Can you work these out from the drawing? Everything is in mm from the part's minimum corner. Round coordinates to 2 decimals unless told otherwise and drop trailing zeros. Order: outer loops, then holes, each group sorted by start corner. A loop starts at its lowest first (then second) coordinate and runs counter-clockwise, first axis right, second up. Notation, with made-up numbers: (74, -21) -> (122, -21) arc R14 cw to (122, 6) -> close; hole circle Ø8 at (12, -1.75). An arc over 180 degrees is marked (long way). One line per item, written item: value.
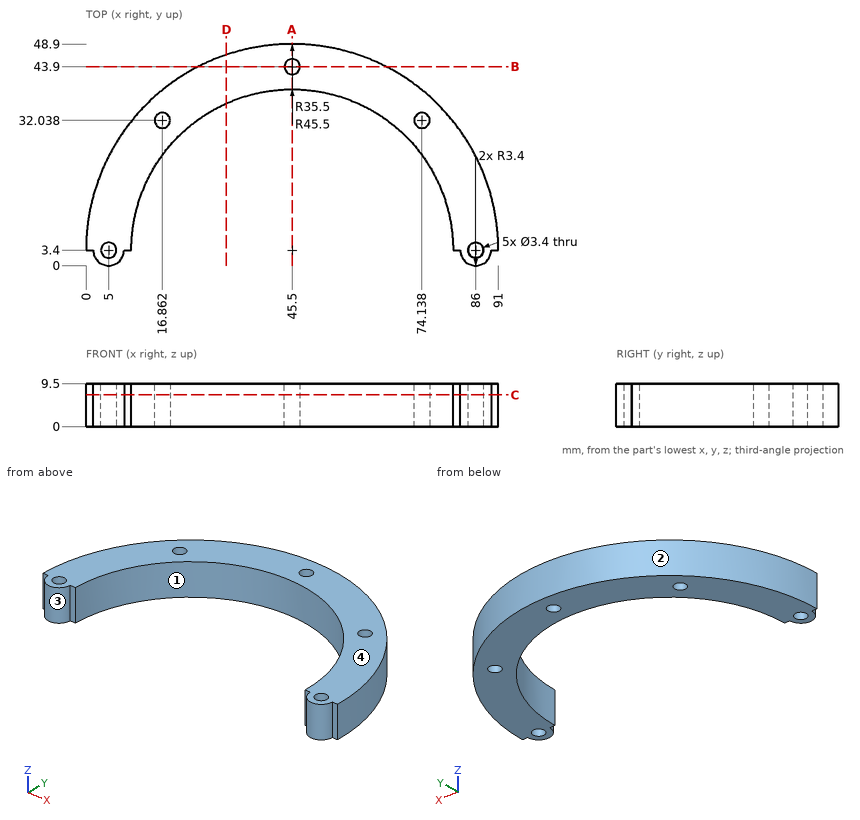
Q1. I want a section at A-A on x = 45.5. List the corners of the cut face in (y, z) for me, plus the area to 3 significant figures.
Answers below:
outline: (38.9, 0) -> (42.2, 0) -> (42.2, 9.5) -> (38.9, 9.5) -> close; (45.6, 0) -> (48.9, 0) -> (48.9, 9.5) -> (45.6, 9.5) -> close
area: 62.7 mm^2
Q2. Please list where these lines run through material, in increasing order: line 1 along Y through (x, z) = (45.5, 2); line 2 along Y through (x, z) = (86, 4) (1 decimal); line 3 along X through (y, z) = (15, 3).
Answers below:
line 1: 38.9 to 42.2, 45.6 to 48.9
line 2: 0 to 1.7, 5.1 to 24.1
line 3: 1.5 to 11.95, 79.05 to 89.5
Q3. I want a section at D-D on x = 31. List the corners of the cut face in (y, z) for me.
Answers below:
outline: (35.8, 0) -> (46.53, 0) -> (46.53, 9.5) -> (35.8, 9.5) -> close
Q4. I want a section at B-B on y = 43.9. List the corners of the cut face in (x, z) for me, plus the area to 3 significant figures.
Answers below:
outline: (24.76, 0) -> (43.8, 0) -> (43.8, 9.5) -> (24.76, 9.5) -> close; (47.2, 0) -> (66.24, 0) -> (66.24, 9.5) -> (47.2, 9.5) -> close
area: 362 mm^2
Q5. Will these pins go through, and if not, where does the flat tip stop? pin 1 Ø2 at (x, z) = (42.5, 6.5) entering from -Y; pin 2 Ø1 at (y, z) = (24.5, 1.5) entering from +X; pin 3 Ø0.5 at (x, z) = (82, 5) entering from -Y.
Answers below:
pin 1: y = 38.67
pin 2: x = 86.07
pin 3: y = 3.4
Q6. We'd pull the mould along X, two halves only. Please class the marked faces 1, 2, 3 and 4: released by +X, released by -X, zero draft, split by the parting line, or undercut.
Answers below:
face 1: undercut
face 2: split by the parting line
face 3: undercut
face 4: zero draft
Q7. I want a section at C-C on z = 7. List the corners of the cut face in (x, y) for me.
Answers below:
outline: (0, 3.4) -> (1.6, 3.4) arc R3.4 ccw to (8.4, 3.4) -> (10, 3.4) arc R35.5 cw to (81, 3.4) -> (82.6, 3.4) arc R3.4 ccw to (89.4, 3.4) -> (91, 3.4) arc R45.5 ccw to start; hole circle Ø3.4 at (5, 3.4); hole circle Ø3.4 at (16.86, 32.04); hole circle Ø3.4 at (45.5, 43.9); hole circle Ø3.4 at (74.14, 32.04); hole circle Ø3.4 at (86, 3.4)
